Part print with two shaded views. Sizes in mm from the minimum x, y, z corner. A direction names the side the tool comes from. Coordinates: 2 decimals unless noted, no trailing zeros. Loops run counter-clockwise (first coordinate to the right, second up) from the corner with the lowest first, then second, coordinate; pieces in that order, holes last.
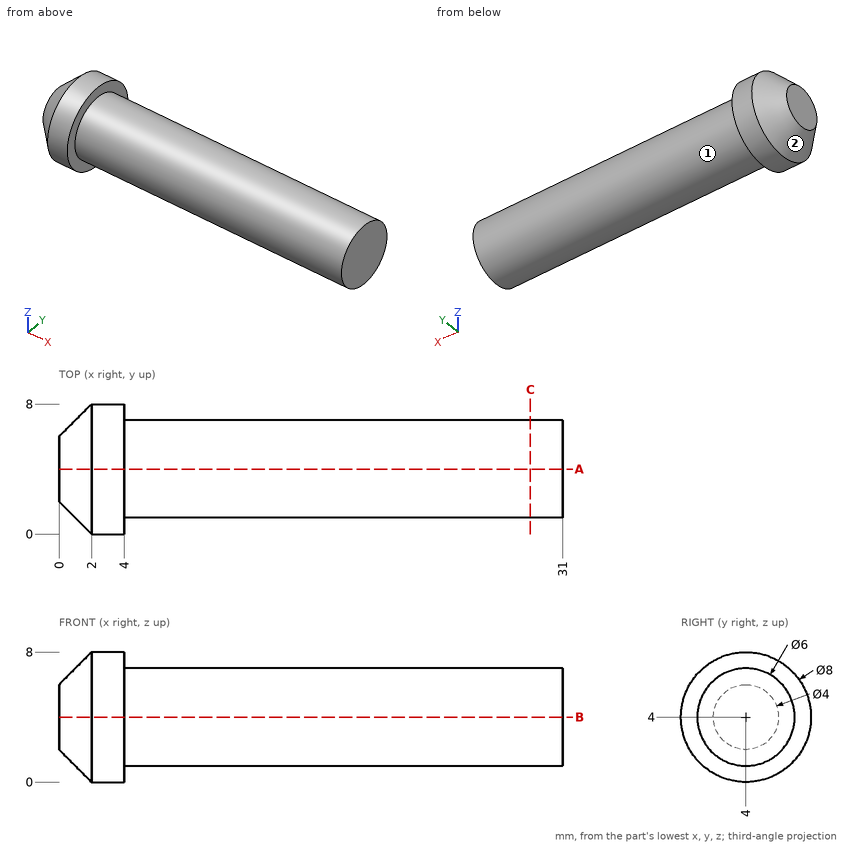
Q1. Flat gauge pins, fed straight in: P1, Ø4, axis at x = 17.5, z = 4.5, coming from the +Y side; P2, Ø2, axis at x = 17, y = 3.5, coming from the -Z side; P3, Ø3, axis at x = 15, y = 6, coming from the +Z side; P4, Ø2, axis at x = 4, y = 3.5, coming from the -Z side. Where does each tip first touch, or does it go through?
Answers:
P1: stops at y = 7
P2: stops at z = 1
P3: stops at z = 6.96
P4: stops at z = 0
Q2. Slice it at A-A (y = 4). List the corners of the cut face in (x, z), and give its area (3 significant figures).
Answers:
outline: (0, 2) - (2, 0) - (4, 0) - (4, 1) - (31, 1) - (31, 7) - (4, 7) - (4, 8) - (2, 8) - (0, 6) - close
area: 190 mm2
Q3. Slice it at C-C (x = 29). List the corners of the cut face in (y, z).
Answers:
outline: circle Ø6 at (4, 4)
Q4. Drill centre lines: line 1 (X direction, y = 7.5, z = 2.5); line 2 (Y direction, x = 25, z = 1.5); line 3 (Y direction, x = 24.5, z = 3.5). Where is each one in solid material? Low to high.
Answers:
line 1: x = 1.81 to 4
line 2: y = 2.34 to 5.66
line 3: y = 1.04 to 6.96
Q5. Which spindle directions (+Z, -Z, +X, -X, +Y, -Y) get a long thin tool onto all of the face, cutting with end or side? Do the marked faces 1 and 2. Say none if no direction does.
Answers:
face 1: +X
face 2: -X
